Model file for the job. Use its own axes, mm. Round coordinates to 2 decimals unless told otherwise and drop trailing zeros. Put each result on its own line as item: value. Start each with the question number.
Q1. Probe L1, parallel to X at y = -43.5, z = 0.8; L2, parallel to Y at x = 52.5, z = 2.2; L3, parallel to X at y = -21, z = 2.4. List the from-to ranges inside material, lowest first.
Q2. Flat gauge pins, fed straight in: P1, Ø2, axis at x = 118.9, y = 13.63, coming from the +Z side; P2, Ø3.5, axis at x = 66.4, y = 2, coming from the -Z side. Where does each tip first touch, or does it go through?
Q3. Pull direction X, two halves, no side cores. Call faces 1 (the face through (24.5, -21, 1)), 2 (the face through (84.9, 2.07, 1.52)), 3 (the face through (126.874, -59.27, 1.479)): released by +X, released by -X, zero draft, split by the parting line, or undercut.
Autodesk Inventor part; units mm, degrees
ref_plane "YZ Plane" through (0, 0, 0) normal (1, 0, 0) x (0, 1, 0)
ref_plane "XZ Plane" through (0, 0, 0) normal (0, 1, 0) x (-1, 0, 0)
ref_plane "XY Plane" through (0, 0, 0) normal (0, 0, 1) x (1, 0, 0)
sketch "Эскиз1" plane through (0, 0, 0) normal (0, 0, 1) x (1, 0, 0)
  circle A0 centre (41.8996, -50.8737) radius 1.5
  circle A1 centre (115.8996, -50.8737) radius 1.5
  line L0 (128.2996, -55.7737) -> (128.2996, 12.0263)
  arc A2 (128.2996, 12.0263) -> (123.2996, 17.0263) centre (123.2996, 12.0263) ccw
  line L1 (123.2996, 17.0263) -> (29.4996, 17.0263)
  arc A3 (29.4996, 17.0263) -> (24.4996, 12.0263) centre (29.4996, 12.0263) ccw
  line L2 (24.4996, 12.0263) -> (24.4996, -55.7737)
  arc A4 (24.4996, -55.7737) -> (29.4996, -60.7737) centre (29.4996, -55.7737) ccw
  line L3 (29.4996, -60.7737) -> (123.2996, -60.7737)
  arc A5 (123.2996, -60.7737) -> (128.2996, -55.7737) centre (123.2996, -55.7737) ccw
  line L4 (53.8996, 12.1263) -> (105.3355, 12.1263)
  arc A6 (105.3355, 9.1263) -> (105.3355, 12.1263) centre (105.3355, 10.6263) ccw
  line L5 (105.3355, 9.1263) -> (53.8996, 9.1263)
  arc A7 (53.8996, 12.1263) -> (53.8996, 9.1263) centre (53.8996, 10.6263) ccw
  circle A8 centre (53.8996, -6.8737) radius 1.5
  circle A9 centre (53.8996, -36.8737) radius 1.5
  circle A10 centre (103.8996, -36.8737) radius 1.5
  circle A11 centre (103.8996, -6.8737) radius 1.5
  circle A12 centre (118.8996, -44.3737) radius 1.375
  circle A13 centre (32.8996, -44.3737) radius 1.375
  circle A14 centre (32.8996, 13.6263) radius 1.375
  circle A15 centre (118.8996, 13.6263) radius 1.375
  line L6 (105.3355, -0.8737) -> (53.8996, -0.8737)
  arc A16 (53.8996, 2.1263) -> (53.8996, -0.8737) centre (53.8996, 0.6263) ccw
  line L7 (53.8996, 2.1263) -> (105.3355, 2.1263)
  arc A17 (105.3355, -0.8737) -> (105.3355, 2.1263) centre (105.3355, 0.6263) ccw
  arc A18 (53.8996, -42.8737) -> (53.8996, -45.8737) centre (53.8996, -44.3737) ccw
  line L8 (53.8996, -42.8737) -> (103.8996, -42.8737)
  arc A19 (103.8996, -45.8737) -> (103.8996, -42.8737) centre (103.8996, -44.3737) ccw
  line L9 (103.8996, -45.8737) -> (53.8996, -45.8737)
  line L10 (103.8996, -55.8737) -> (53.8996, -55.8737)
  arc A20 (53.8996, -52.8737) -> (53.8996, -55.8737) centre (53.8996, -54.3737) ccw
  line L11 (53.8996, -52.8737) -> (103.8996, -52.8737)
  arc A21 (103.8996, -55.8737) -> (103.8996, -52.8737) centre (103.8996, -54.3737) ccw
  line L12 (76.7782, -31.8737) -> (72.5356, -27.6311)
  arc A22 (74.6569, -25.5097) -> (72.5356, -27.6311) centre (73.5963, -26.5704) ccw
  line L13 (74.6569, -25.5097) -> (77.3996, -28.2524)
  line L14 (77.3996, -28.2524) -> (77.3996, -11.8737)
  arc A23 (80.3996, -11.8737) -> (77.3996, -11.8737) centre (78.8996, -11.8737) ccw
  line L15 (80.3996, -11.8737) -> (80.3996, -28.2524)
  line L16 (80.3996, -28.2524) -> (83.1422, -25.5097)
  arc A24 (85.2635, -27.6311) -> (83.1422, -25.5097) centre (84.2029, -26.5704) ccw
  line L17 (85.2635, -27.6311) -> (81.0209, -31.8737)
  arc A25 (76.7782, -31.8737) -> (81.0209, -31.8737) centre (78.8996, -31.8737) ccw
  point P0 (0, 0)
extrude "Выдавливание1" add sketch "Эскиз1" along normal blind 3 contours A0 | A1 | A5 L3 A4 L2 A3 L1 A2 L0 | L4 A6 L5 A7 | A8 | A9 | A10 | A11 | L6 A16 L7 A17 | L8 A19 L9 A18 | L10 A20 L11 A21 | L12 A22 L13 L14 A23 L15 L16 A24 L17 A25
sketch "Эскиз2" plane through (0, 0, 3) normal (0, 0, 1) x (1, 0, 0)
  line L0 (29.4996, -60.7737) -> (123.2996, -60.7737)
  circle A0 centre (51.3996, -43.2737) radius 1.5
  circle A1 centre (101.3996, -43.2737) radius 1.5
  point P0 (0, 0)
  dimension "d6" = 3
  dimension "d7" = 3
extrude "Выдавливание2" cut sketch "Эскиз2" against normal blind 3
sketch "Эскиз3" plane through (0, 0, 3) normal (0, 0, 1) x (1, 0, 0)
  line L0 (24.4996, 12.0263) -> (24.4996, -55.7737)
  line L1 (24.4996, -21.8737) -> (128.2996, -21.8737)
  line L2 (128.2996, -55.7737) -> (128.2996, 12.0263)
  line L3 (76.3996, -21.8737) -> (76.3996, 17.0263)
  line L4 (123.2996, 17.0263) -> (29.4996, 17.0263)
  circle A0 centre (118.8996, -44.3737) radius 1.375
  circle A1 centre (101.3996, -43.2737) radius 1.5
  circle A2 centre (51.3996, -20.4987) radius 1.5
  circle A3 centre (101.3996, -20.4987) radius 1.5
  line L5 (76.3996, -20.4987) -> (76.3996, -7.9987)
  line L6 (76.3996, -7.9987) -> (76.3996, 2.0013)
  circle A4 centre (66.3996, 2.0013) radius 1.5
  circle A5 centre (86.3996, 2.0013) radius 1.5
  point P0 (0, 0)
  point P1 (101.999, -21.8737)
  point P2 (100.8001, -21.8737)
  dimension "d13" = 3
  dimension "d14" = 3
  dimension "d19" = 3
  dimension "d20" = 3
extrude "Выдавливание3" cut sketch "Эскиз3" against normal blind 3 contours A2 L1 | A3 L1 | L1 A2 | A4 | A5 picked at (100.9144, -20.3462)
properties part number "down_plate"
Ans:
1. L1: x = 24.5 to 31.84, 33.96 to 49.92, 52.88 to 99.92, 102.88 to 117.84, 119.96 to 128.3
1. L2: y = -60.77 to -44.29, -42.25 to -21.52, -19.48 to 17.03
1. L3: x = 24.5 to 49.99, 52.81 to 99.99, 102.81 to 128.3
2. P1: passes through
2. P2: stops at z = 0
3. face 1: released by -X
3. face 2: undercut
3. face 3: released by +X
